Part model, mm, in its own coordinate system. A direction names the side the tool comes from. Give positions to 0.01 mm unless a question says otherwise; leave off trailing zeros. Write each loop counter-clockwise with the first axis right and the second up, starting at its lowest first coordinate (ties: lowest second). Pieces come first, ordered by that corner, then holes.
```python
from build123d import *

# Parameters (mm, degrees)
F0_R     = 4
F1_DEPTH = 12
F5_DEPTH = 25


with BuildPart() as f1:
    # F0 (on Top) → F1 (new body)
    with BuildSketch(Plane.XY):
        with BuildLine():
            ThreePointArc((-26.0048357101, 50.7444812044), (-29.3644274881, 53.2410792158), (-31.4666877274, 56.8605212214))
            ThreePointArc((-31.4666877274, 56.8605212214), (-40.0213923063, 62.999974576), (-48.5468142888, 56.8199229623))
            ThreePointArc((-48.5468142888, 56.8199229623), (-49.9581514965, 53.9510477252), (-52.1002110708, 51.5774642275))
            Line((-52.1002110708, 51.5774642275), (-64.5975648535, 41.0909392778))
            ThreePointArc((-64.5975648535, 41.0909392778), (-70.7961493932, 33.0127866299), (-73, 23.0718589569))
            Line((-73, 23.0718589569), (-73, 6.7840487521))
            ThreePointArc((-73, 6.7840487521), (-73.7491959701, 2.5215841304), (-75.9069767442, -1.2299330805))
            ThreePointArc((-75.9069767442, -1.2299330805), (-75.0048915598, -13.7038255761), (-62.5073050486, -13.2325686734))
            ThreePointArc((-62.5073050486, -13.2325686734), (-59.8003263562, -11.7702356961), (-56.747924728, -12.1562352786))
            Line((-56.747924728, -12.1562352786), (-30.1383846638, -24.5644675905))
            ThreePointArc((-30.1383846638, -24.5644675905), (-27.3013538285, -26.880356732), (-25.9102142317, -30.2681018667))
            ThreePointArc((-25.9102142317, -30.2681018667), (-20.3937217432, -37.3356255152), (-11.5094179528, -36.1311646162))
            ThreePointArc((-11.5094179528, -36.1311646162), (-8.6282643598, -34.7280777032), (-5.4272064645, -34.5766601914))
            ThreePointArc((-5.4272064645, -34.5766601914), (30.4444426556, -17.2666126206), (26.8895951939, 22.4042333122))
            ThreePointArc((26.8895951939, 22.4042333122), (25.241110657, 25.4802972467), (24.9393792274, 28.9571677853))
            ThreePointArc((24.9393792274, 28.9571677853), (20.8346498039, 37.591189714), (11.2748155965, 37.6598062869))
            ThreePointArc((11.2748155965, 37.6598062869), (7.2373944377, 36.3866405331), (3.0794263015, 37.1822670966))
            Line((3.0794263015, 37.1822670966), (-26.0048357101, 50.7444812044))
        make_face()
        with Locations((-69, -7)):
            Circle(F0_R, mode=Mode.SUBTRACT)
        with Locations((-17, -29)):
            Circle(F0_R, mode=Mode.SUBTRACT)
        with BuildLine():
            ThreePointArc((9.72022002, 20.8450791018), (20.8450791018, -9.72022002), (-9.72022002, -20.8450791018))
            Line((-9.72022002, -20.8450791018), (-54.4226364125, 0))
            ThreePointArc((-54.4226364125, 0), (-59.2159612375, 4.203633051), (-61, 10.3243927587))
            Line((-61, 10.3243927587), (-61, 22.8490752496))
            ThreePointArc((-61, 22.8490752496), (-59.8756934444, 27.9204943905), (-56.7134513162, 32.041608567))
            Line((-56.7134513162, 32.041608567), (-43.5116564926, 43.1192297344))
            ThreePointArc((-43.5116564926, 43.1192297344), (-41.4626108227, 44.0208314074), (-39.2500330069, 43.6802831101))
            Line((-39.2500330069, 43.6802831101), (9.72022002, 20.8450791018))
        make_face(mode=Mode.SUBTRACT)
        with Locations((-40, 54)):
            Circle(F0_R, mode=Mode.SUBTRACT)
        with Locations((16, 30)):
            Circle(F0_R, mode=Mode.SUBTRACT)
        with BuildLine():
            Line((-54.4226364125, 0), (-9.72022002, -20.8450791018))
            ThreePointArc((-9.72022002, -20.8450791018), (20.8450791018, -9.72022002), (9.72022002, 20.8450791018))
            Line((9.72022002, 20.8450791018), (-39.2500330069, 43.6802831101))
            ThreePointArc((-39.2500330069, 43.6802831101), (-41.4626108227, 44.0208314074), (-43.5116564926, 43.1192297344))
            Line((-43.5116564926, 43.1192297344), (-56.7134513162, 32.041608567))
            ThreePointArc((-56.7134513162, 32.041608567), (-59.8756934444, 27.9204943905), (-61, 22.8490752496))
            Line((-61, 22.8490752496), (-61, 10.3243927587))
            ThreePointArc((-61, 10.3243927587), (-59.2159612375, 4.203633051), (-54.4226364125, 0))
        make_face()
    extrude(amount=F1_DEPTH)

    # F3 (on offset) → F5 (cut)
    with BuildSketch(Plane.XY.offset(12)):
        with BuildLine():
            Line((9.72022002, 20.8450791018), (-30.6963252268, 39.6916236666))
            ThreePointArc((-30.6963252268, 39.6916236666), (-61.2616243486, 28.5667645848), (-50.1367652668, -1.9985345371))
            Line((-50.1367652668, -1.9985345371), (-9.72022002, -20.8450791018))
            ThreePointArc((-9.72022002, -20.8450791018), (20.8450791018, -9.72022002), (9.72022002, 20.8450791018))
        make_face()
    extrude(amount=-F5_DEPTH, mode=Mode.SUBTRACT)


solid = f1.part
```
1) Saw through at B-B, the plane y = -29. Write the cut outline in (x, z).
Answers follow:
outline: (-26.21, 0) - (-21, 0) - (-21, 12) - (-26.21, 12) - close; (-13, 0) - (19.6, 0) - (19.6, 12) - (-13, 12) - close
2) 3-axis set-ups, long thin cutter, end or side, ignore diameter. For faces 1 (the face through (-27.33, -26.84, 5.92)), 2 (the face through (-43.629, -18.273, 5.916)), 3 (the face through (-10.21, 30.14, 6.08)): which of +Z, -Z, +X, -X, +Y, -Y reach the whole face in a straight line?
Answers follow:
face 1: +Z, -Z, -X, -Y
face 2: +Z, -Z, -Y
face 3: +Z, -Z
3) Wall check: L1, parallel to Y at x = -40, z = 3; L2, parallel to Y at x = -19, z = 9.5; L3, parallel to X at y = -15, z = 5.75. Give the ranges that are in metal, low to high.
Answers follow:
L1: y = -19.97 to -6.73, 41.84 to 50, 58 to 63
L2: y = -37.77 to -32.46, -25.54 to -16.52, 34.24 to 47.48
L3: x = -73.12 to -64.88, -50.65 to -22.26, 17.44 to 31.62
4) Saw through at C-C, the plane y = -7. Write the cut outline in (x, z), then the cut area to 3 significant figures.
Answers follow:
outline: (-78, 0) - (-73, 0) - (-73, 12) - (-78, 12) - close; (-65, 0) - (-39.41, 0) - (-39.41, 12) - (-65, 12) - close; (21.91, 0) - (34.29, 0) - (34.29, 12) - (21.91, 12) - close
area: 516 mm2
5) Pin check, flat tips, straight feed: pin 1 Ø1 at (x, z) = (-13.5, 10.5) entering from +Y; pin 2 Ø6 at (y, z) = (43, 9) entering from +X; pin 3 Ø1.5 at (x, z) = (5, 8.5) entering from +Y. Stop position of each tip, or through.
Answers follow:
pin 1: stops at y = 45.15
pin 2: stops at x = -2.96
pin 3: stops at y = 36.74
6) Two-plate mould, pull along Y, no slides. Class faces 4 (the face through (-11.26, 43.87, 5.92)), 5 (the face through (-22, -17, 12)), 6 (the face through (20.626, -10.176, 6.084)): +Y half, -Y half, draft (parallel to the pull), parting line (faces both ways), or undercut.
Answers follow:
face 4: +Y half
face 5: draft
face 6: undercut
7) Saw through at D-D, the plane x = -54. Write the cut outline in (y, z).
Answers follow:
outline: (-13.44, 0) - (0.29, 0) - (0.29, 12) - (-13.44, 12) - close; (37.41, 0) - (49.98, 0) - (49.98, 12) - (37.41, 12) - close
8) Saw through at A-A, the plane x = -17. Write the cut outline in (y, z).
Answers follow:
outline: (-38, 0) - (-33, 0) - (-33, 12) - (-38, 12) - close; (-25, 0) - (-17.45, 0) - (-17.45, 12) - (-25, 12) - close; (33.3, 0) - (46.55, 0) - (46.55, 12) - (33.3, 12) - close
